Geometry: final body of the model. Coordinates: model frame, mm. Coordinates: 2 decimals unless noted, no trailing zeros. Write each loop counter-clockwise with the first axis right and the second up, starting at its lowest first coordinate (ties: lowest second). Pieces come first, ordered by that corner, then holes. Notation, with made-up numbers: (43.5, 16.25) - (52.5, 16.25) arc R8 ccw to (52.5, 23.25) - close; hole circle Ø4 at (-11.75, -35). An arc over 180 degrees is marked (long way). Answer as a JSON object with one key per item and string values. Group by question number.
Item 1: Line query: line 1 along Y through (x, z) = (1.25, 2.75); line 2 along Z through (x, y) = (5.25, -11); line 3 along X through (y, z) = (1, 4.75). Output: solid intervals per line, ascending. Write a range as from..to.
Item 2: Section D-D on y = 4. Return loops of the section in (x, z), and give its area (3 significant figures).
Item 3: Mould query, pull axis Y, two halves, no side actions, for faces 1 (the flat face through (-5.55, -11.83, 2.97)), 2 (the flat face through (0, -6, 0)), 3 (the cylindrical face through (-1.5, 0.07, 2.96)), 4 (the cylindrical face through (-0.195, -22.513, 2.958)). Classes: pulls with the +Y half, pulls with the -Y half, needs draft (parallel to the pull), parting line crosses it, or undercut.
Item 4: Section C-C on z = 3.5. Return loops of the section in (x, y) (3 decimals).
Item 5: First-contact query: pin 1 Ø2 at (y, z) = (1.5, 1) entering from -X; pin 2 Ø3 at (y, z) = (-18, 3) entering from +X. Flat tips, straight axial feed; report the tip coordinate or a pass-through.
Item 6: Section A-A on x = 0. Return loops of the section in (y, z) (3 decimals), and give its area (3 significant figures).
Item 7: Section B-B on y = -25. Return loops of the section in (x, z).
```python
from build123d import *

# Parameters (mm, degrees)
SKETCH_R    = 1.5
PAD_DEPTH   = 6
FILLET_R    = 1
FILLET001_R = 1
FILLET002_R = 1
FILLET003_R = 1


with BuildPart() as part:
    # Sketch → Pad (new body)
    with BuildSketch(Plane.XY):
        with BuildLine():
            Line((-7.325, 0), (-3.725, -24))
            ThreePointArc((-3.725, -24), (0, -27.725), (3.725, -24))
            Line((7.325, 0), (3.725, -24))
            ThreePointArc((7.325, 0), (0, 7.325), (-7.325, 0))
        make_face()
        Circle(SKETCH_R, mode=Mode.SUBTRACT)
        with Locations((0, -24)):
            Circle(SKETCH_R, mode=Mode.SUBTRACT)
    extrude(amount=PAD_DEPTH)

    # Fillet
    fillet_edges = [part.edges().sort_by_distance(p)[0] for p in [
        (-5.525, -12, 6),
    ]]
    fillet(fillet_edges, radius=FILLET_R)

    # Fillet001
    fillet001_edges = [part.edges().sort_by_distance(p)[0] for p in [
        (5.525, -12, 6),
    ]]
    fillet(fillet001_edges, radius=FILLET001_R)

    # Fillet002
    fillet002_edges = [part.edges().sort_by_distance(p)[0] for p in [
        (-5.525, -12, 0),
    ]]
    fillet(fillet002_edges, radius=FILLET002_R)

    # Fillet003
    fillet003_edges = [part.edges().sort_by_distance(p)[0] for p in [
        (5.525, -12, 0),
    ]]
    fillet(fillet003_edges, radius=FILLET003_R)


solid = part.part
```
Checks:
{
 "1": {"line 1": "-27.51..-24.83, -23.17..-0.83, 0.83..7.22", "line 2": "0.19..5.81", "line 3": "-7.26..-1.12, 1.12..7.26"},
 "2": {"outline": "(-6.14, 0) - (6.14, 0) - (6.14, 6) - (-6.14, 6) - close", "area": "73.6 mm^2"},
 "3": {"face 1": "pulls with the -Y half", "face 2": "needs draft", "face 3": "undercut", "face 4": "undercut"},
 "4": {"outline": "(-7.325, 0) - (-3.725, -24) arc R3.725 ccw to (3.725, -24) - (7.325, 0) arc R7.325 ccw to start; hole circle Ø3 at (0, -24); hole circle Ø3 at (0, 0)"},
 "5": {"pin 1": "x = -7.31", "pin 2": "x = 4.85"},
 "6": {"outline": "(-27.725, 0) - (-25.5, 0) - (-25.5, 6) - (-27.725, 6) - close; (-22.5, 0) - (-1.5, 0) - (-1.5, 6) - (-22.5, 6) - close; (1.5, 0) - (7.325, 0) - (7.325, 6) - (1.5, 6) - close", "area": "174 mm^2"},
 "7": {"outline": "(-3.59, 0) - (-1.12, 0) - (-1.12, 6) - (-3.59, 6) - close; (1.12, 0) - (3.59, 0) - (3.59, 6) - (1.12, 6) - close"}
}
